Input: part model. Units: mm. Frame: model coordinates. Face numbers are marked on the shaded views. A direction names the side the tool comes from. Coordinates: 2 decimals unless noted, no trailing zeros. Loops run counter-clockwise (first coordinate to the right, second up) from the corner with the lowest first, then second, coordinate; pieces in that order, holes last. Notation, with made-up numbers: M -28.5,9.25 L -18.5,9.25 A27 ccw -18.5,36.25 Z; hole C 70,81.5 d8. An arc over 180 degrees is marked long. Use a Markdown table: item, result. Add a question column.
1. Section A-A on z = 0. Output: boundary loops of the cut face in (x, y).
2. Pin query (flat end, axial travel): pin 1 (3 mm diameter, centred on x = 0.5, z = 6, fed in from -Y); pin 2 (5.5 mm diameter, centred on y = 2.5, z = -1.5, fed in from +X); pin 3 (1 mm diameter, centred on x = -4, y = -7.5, fed in from +Z); pin 4 (2.5 mm diameter, centred on x = 6, y = 0.5, fed in from -Z). Return the tip coordinate at first contact, or that it passes through.
3. Line query: L1, parallel to Y at x = 0.5, z = 0; L2, parallel to X at y = -8, z = -1.5; L3, parallel to X at y = 1.5, z = -8.5. Output: solid intervals per line, ascending. Write a range as [from, to].
4. Section D-D on x = 0.5. Output: boundary loops of the cut face in (y, z).
5. Section B-B on y = 0. Output: boundary loops of the cut face in (x, z), then the cut area to 3 significant figures.
6. Draft query along X for the marked faces 1, 2 and 3. Return one class per face: +X half, -X half, draft (parallel to the pull), parting line (faces both ways), or undercut.
7. Set-up query: the marked faces 4, 5 and 6. Return all of +Z, -Z, +X, -X, +Y, -Y with unobstructed straight access to the full face (end or side cutting, diameter ignored); none if empty.
8. Section C-C on x = 4.5. Output: boundary loops of the cut face in (y, z), then the cut area to 3 significant figures.
```python
from build123d import *

# Parameters (mm, degrees)
SKETCH1_R           = 6.4643
BOSS_EXTRUDE1_DEPTH = 6.8707
SKETCH2_R           = 12.068907195
SKETCH2_R_2         = 7.4295
CUT_EXTRUDE1_DEPTH  = 13.7414
BOSS_EXTRUDE3_START = -4.445
SKETCH3_R           = 6.4643
BOSS_EXTRUDE3_DEPTH = 4.445
SKETCH4_R           = 13.191665885
SKETCH4_R_2         = 8.4455
CUT_EXTRUDE2_DEPTH  = 1.651
CHAMFER1_SIZE       = 0.254


with BuildPart() as part:
    # Sketch1 → Boss-Extrude1 (new, symmetric)
    with BuildSketch(Plane(origin=(0, 0, 0), x_dir=(0, 0, -1), z_dir=(1, 0, 0))):
        with BuildLine():
            Line((-7.47395, 4.000479841), (-7.47395, -4.000479841))
            ThreePointArc((-7.47395, -4.000479841), (0, -8.47725), (7.47395, -4.000479841))
            Line((7.47395, -4.000479841), (7.47395, 4.000479841))
            ThreePointArc((7.47395, 4.000479841), (0, 8.47725), (-7.47395, 4.000479841))
        make_face()
        Circle(SKETCH1_R, mode=Mode.SUBTRACT)
    extrude(amount=BOSS_EXTRUDE1_DEPTH, both=True)

    # Sketch2 → Cut-Extrude1 (cut)
    with BuildSketch(Plane(origin=(3.5179, 0, 0), x_dir=(0, 0, -1), z_dir=(1, 0, 0))):
        Circle(SKETCH2_R)
        Circle(SKETCH2_R_2, mode=Mode.SUBTRACT)
    extrude(amount=-CUT_EXTRUDE1_DEPTH, mode=Mode.SUBTRACT)

    # Sketch3 → Boss-Extrude3 (add)
    with BuildSketch(Plane(origin=(-2.4257, 0, 0), x_dir=(0, 0, -1), z_dir=(1, 0, 0)).offset(BOSS_EXTRUDE3_START)):
        with BuildLine():
            ThreePointArc((-0.831056545, 9.488675883), (-6.735192091, 6.735192091), (-9.488675883, 0.831056545))
            ThreePointArc((-9.488675883, 0.831056545), (-8.69315, 0), (-9.488675883, -0.831056545))
            ThreePointArc((-9.488675883, -0.831056545), (-6.735192091, -6.735192091), (-0.831056545, -9.488675883))
            ThreePointArc((-0.831056545, -9.488675883), (0, -8.69315), (0.831056545, -9.488675883))
            ThreePointArc((0.831056545, -9.488675883), (6.735192091, -6.735192091), (9.488675883, -0.831056545))
            ThreePointArc((9.488675883, -0.831056545), (8.69315, 0), (9.488675883, 0.831056545))
            ThreePointArc((9.488675883, 0.831056545), (6.735192091, 6.735192091), (0.831056545, 9.488675883))
            ThreePointArc((0.831056545, 9.488675883), (0, 8.69315), (-0.831056545, 9.488675883))
        make_face()
        Circle(SKETCH3_R, mode=Mode.SUBTRACT)
    extrude(amount=BOSS_EXTRUDE3_DEPTH)

    # Sketch4 → Cut-Extrude2 (cut)
    with BuildSketch(Plane(origin=(-2.4257, 0, 0), x_dir=(0, 0, -1), z_dir=(1, 0, 0))):
        Circle(SKETCH4_R)
        Circle(SKETCH4_R_2, mode=Mode.SUBTRACT)
    extrude(amount=-CUT_EXTRUDE2_DEPTH, mode=Mode.SUBTRACT)

    # Chamfer1
    chamfer1_edges = [part.edges().sort_by_distance(p)[0] for p in [
        (-4.0767, 6.735192091, -6.735192091),
        (-4.0767, 6.735192091, 6.735192091),
        (-4.0767, -6.735192091, -6.735192091),
        (-4.0767, -6.735192091, 6.735192091),
    ]]
    chamfer(chamfer1_edges, length=CHAMFER1_SIZE)


solid = part.part
```
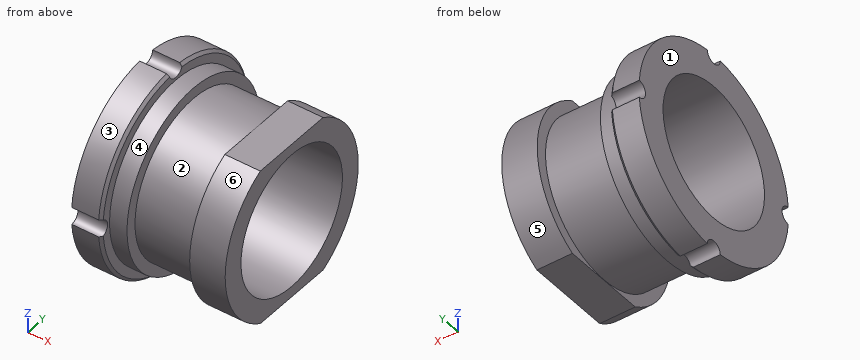
Answers below:
| question | item | result |
|---|---|---|
| 1 | outline | M -6.87,-8.69 L -4.08,-8.69 L -4.08,-8.45 L -2.43,-8.45 L -2.43,-7.43 L 3.52,-7.43 L 3.52,-8.48 L 6.87,-8.48 L 6.87,-6.46 L -6.87,-6.46 Z; M -6.87,6.46 L 6.87,6.46 L 6.87,8.48 L 3.52,8.48 L 3.52,7.43 L -2.43,7.43 L -2.43,8.45 L -4.08,8.45 L -4.08,8.69 L -6.87,8.69 Z |
| 2 | pin 1 | stops at y = -5.91 |
| 2 | pin 2 | passes through |
| 2 | pin 3 | stops at z = 6.32 |
| 2 | pin 4 | stops at z = -7.47 |
| 3 | L1 | y = [-7.43, -6.46], [6.46, 7.43] |
| 3 | L2 | x = [-6.87, -2.43], [3.52, 6.87] |
| 3 | L3 | x = [-6.87, -4.08] |
| 4 | outline | C 0,0 d14.86; hole C 0,0 d12.93 |
| 5 | outline | M -6.87,-8.69 L -4.08,-8.69 L -4.08,-8.45 L -2.43,-8.45 L -2.43,-7.43 L 3.52,-7.43 L 3.52,-7.47 L 6.87,-7.47 L 6.87,-6.46 L -6.87,-6.46 Z; M -6.87,6.46 L 6.87,6.46 L 6.87,7.47 L 3.52,7.47 L 3.52,7.43 L -2.43,7.43 L -2.43,8.45 L -4.08,8.45 L -4.08,8.69 L -6.87,8.69 Z |
| 5 | area | 37.2 mm² |
| 6 | face 1 | -X half |
| 6 | face 2 | undercut |
| 6 | face 3 | draft |
| 7 | face 4 | none |
| 7 | face 5 | +X, +Y |
| 7 | face 6 | +X, -Y |
| 8 | outline | M -4,-7.47 L 4,-7.47 A8.48 ccw 4,7.47 L -4,7.47 A8.48 ccw Z; hole C 0,0 d12.93 |
| 8 | area | 83.7 mm² |
